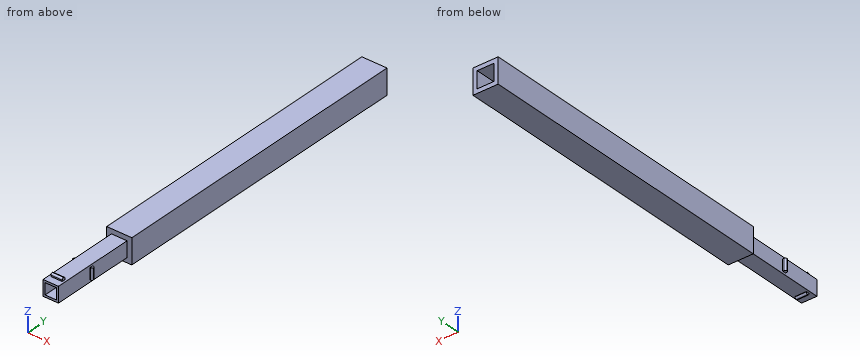
Autodesk Inventor part; units mm, degrees
ref_plane "YZ Plane" through (0, 0, 0) normal (1, 0, 0) x (0, 1, 0)
ref_plane "XZ Plane" through (0, 0, 0) normal (0, 1, 0) x (-1, 0, 0)
ref_plane "XY Plane" through (0, 0, 0) normal (0, 0, 1) x (1, 0, 0)
sketch "Szkic1" plane through (0, 0, 0) normal (0, 1, 0) x (-1, 0, 0)
  line L0 (0, 0) -> (12, 0)
  line L1 (12, 0) -> (12, -12)
  line L2 (12, -12) -> (0, -12)
  line L3 (0, -12) -> (0, 0)
  dimension "d0" = 12
  dimension "d1" = 12
extrude "Wyciągnięcie proste1" add sketch "Szkic1" along normal blind 86
sketch "Szkic2" plane through (0, 86, 0) normal (0, 1, 0) x (1, 0, 0)
  line L0 (0, 12) -> (-12, 12)
  line L1 (-12, 12) -> (-12, 0)
  line L2 (-12, 0) -> (0, 0)
  line L3 (0, 0) -> (0, 12)
  line L4 (-10, 2) -> (-10, 10)
  line L5 (-10, 10) -> (-2, 10)
  line L6 (-2, 10) -> (-2, 2)
  line L7 (-2, 2) -> (-10, 2)
  dimension "d4" = 2
extrude "Wyciągnięcie proste2" cut sketch "Szkic2" against normal blind 86 contours L4 L5 L6 L7
sketch "Szkic9" plane through (0, 0, 0) normal (0, -1, 0) x (1, 0, 0)
  line L0 (-2, -10) -> (-10, -10)
  line L1 (-2, -2) -> (-2, -10)
  line L2 (-10, -2) -> (-2, -2)
  line L3 (-10, -10) -> (-10, -2)
  line L4 (-2.3, -2.3) -> (-2.3, -9.7)
  line L5 (-2.3, -9.7) -> (-9.7, -9.7)
  line L6 (-9.7, -9.7) -> (-9.7, -2.3)
  line L7 (-9.7, -2.3) -> (-2.3, -2.3)
  line L8 (-3.3, -3.3) -> (-3.3, -8.7)
  line L9 (-3.3, -8.7) -> (-8.7, -8.7)
  line L10 (-8.7, -8.7) -> (-8.7, -3.3)
  line L11 (-8.7, -3.3) -> (-3.3, -3.3)
  point P0 (0, 0)
  dimension "d21" = 0.3
  dimension "d22" = 1
extrude "Wyciągnięcie proste8" add sketch "Szkic9" along normal blind 40 contours L4 L5 L6 L7
sketch "Szkic10" plane through (0, 0, 0) normal (0, 1, 0) x (1, 0, 0)
  line L0 (-2, 2) -> (-2, 10)
  line L1 (-10.1182, 1.9087) -> (-2, 1.9087)
  line L2 (-2, 1.9087) -> (-2, 10)
  line L3 (-2, 10) -> (-10.1182, 10)
  line L4 (-10.1182, 10) -> (-10.1182, 1.9087)
  line L5 (-3.3, 3.3) -> (-3.3, 8.7)
  line L6 (-8.7, 3.3) -> (-3.3, 3.3)
  line L7 (-8.7, 8.7) -> (-8.7, 3.3)
  line L8 (-3.3, 8.7) -> (-8.7, 8.7)
  line L9 (-8.7, 3.3) -> (-3.3, 3.3)
  line L10 (-3.3, 3.3) -> (-3.3, 8.7)
  line L11 (-3.3, 8.7) -> (-8.7, 8.7)
  line L12 (-8.7, 8.7) -> (-8.7, 3.3)
  point P0 (0, 0)
extrude "Wyciągnięcie proste9" add sketch "Szkic10" along normal blind 2
sketch "Szkic11" plane through (-9.7, 0, -9.7) normal (-1, 0, 0) x (0, 0, 1)
  line L0 (7.4, 0) -> (0, 0)
  line L1 (2.1159, 0) -> (2.1159, -20)
  line L2 (1, 2) -> (1, -40)
  line L3 (6.4, 2) -> (6.4, -40)
  line L4 (1, -20) -> (6.4, -20)
  line L5 (6.4, -20) -> (6.4, -21.6)
  line L6 (6.4, -21.6) -> (1, -21.6)
  line L7 (1, -21.6) -> (1, -20)
  point P0 (9.7, 0)
  point P1 (1, -21.6)
  dimension "d27" = 20
  dimension "d28" = 1.6
extrude "Wyciągnięcie proste10" add sketch "Szkic11" along normal blind 1.4 contours L3 L6 L2 L4
pattern_linear "Szyk prostokątny1" count 2 spacing 8.4 along (1, 0, 0) of "Wyciągnięcie proste10"
sketch "Szkic12" plane through (-9.7, 0, -2.3) normal (0, 0, 1) x (1, 0, 0)
  line L0 (9.7, 0) -> (-2.3, 0)
  line L1 (2.9125, 0) -> (2.9125, -35)
  line L2 (1, 2) -> (1, -40)
  line L3 (1, 2) -> (1, -40)
  line L4 (6.4, 2) -> (6.4, -40)
  line L5 (1, -35) -> (6.4, -35)
  line L6 (6.4, -35) -> (6.4, -36.6)
  line L7 (6.4, -36.6) -> (1, -36.6)
  line L8 (1, -36.6) -> (1, -35)
  dimension "d34" = 35
  dimension "d35" = 1.6
extrude "Wyciągnięcie proste11" add sketch "Szkic12" along normal blind 1.4 contours L4 L7 L2 L5
pattern_linear "Szyk prostokątny2" count 2 spacing 8.4 along (0, 0, -1) of "Wyciągnięcie proste11"
fillet "Zaokrąglenie1" radius 2 4 edges at (-8.7, 2, -6) (-6, 2, -3.3) (-6, 2, -8.7) (-3.3, 2, -6)
sketch "Szkic13" plane through (0, 86, 0) normal (0, 1, 0) x (1, 0, 0)
  line L0 (0, 0) -> (0, 12)
  line L1 (-12, 12) -> (-12, 0)
  line L2 (0, 0) -> (-12, 0)
  line L3 (-12, 0) -> (-12, 12)
  line L4 (-12, 12) -> (0, 12)
  line L5 (0, 12) -> (0, 0)
  line L6 (-2, 10) -> (-2, 2)
  line L7 (-10, 2) -> (-10, 10)
  line L8 (-2, 2) -> (-10, 2)
  line L9 (-10, 2) -> (-10, 10)
  line L10 (-10, 10) -> (-2, 10)
  line L11 (-2, 10) -> (-2, 2)
extrude "Wyciągnięcie proste12" add sketch "Szkic13" along normal blind 63
fillet "Zaokrąglenie2" radius 0.8 8 edges at (-11.1, -20, -6) (-11.1, -21.6, -6) (-1.3, -20, -6) (-1.3, -21.6, -6) (-6, -36.6, -0.9) (-6, -35, -0.9) (-6, -35, -10.7) (-6, -36.6, -10.7)
CAD build for the part. Positions are in the model's coordinates, mm. Round coordinates to 2 decimals unless told otherwise and drop trailing zeros. Write each loop counter-clockwise with the first axis right and the second up, starting at its lowest first coordinate (ties: lowest second). Pieces come first, ordered by that corner, then holes.
Item 1: Drill centre lines: L1, parallel to Z at x = -4.5, y = 26.5; L2, parallel to Y at x = -10.5, z = -8.25. Where is each one in solid material? Low to high.
Filled in:
L1: z = -12 to -10, -2 to 0
L2: y = -21.57 to -20.03, 0 to 149
Item 2: Band-saw the part on A-A on y = 59.5. Write the cut outline in (x, z), then the cut area to 3 significant figures.
Filled in:
outline: (-12, -12) - (0, -12) - (0, 0) - (-12, 0) - close; hole (-10, -10) - (-2, -10) - (-2, -2) - (-10, -2) - close
area: 80.0 mm2
Item 3: Drop flat-ended pins along their axis: pin 1 Ø4 at (x, y) = (-6.5, 50) entering from +Z; pin 2 Ø1.1 at (y, z) = (-36, -10) entering from -X; pin 3 Ø1.6 at (x, y) = (-5, -23) entering from +Z; pin 4 Ø1.1 at (y, z) = (-35.5, -1.5) entering from +X. Give the stop position or say it passes through.
Filled in:
pin 1: stops at z = 0
pin 2: stops at x = -9.7
pin 3: stops at z = -2.3
pin 4: stops at x = -3.3
Item 4: Band-saw the part on D-D on y = -25.5. Write the cut outline in (x, z), then the cut area to 3 significant figures.
Filled in:
outline: (-9.7, -9.7) - (-2.3, -9.7) - (-2.3, -2.3) - (-9.7, -2.3) - close; hole (-8.7, -8.7) - (-3.3, -8.7) - (-3.3, -3.3) - (-8.7, -3.3) - close
area: 25.6 mm2
